Could you check a few things on this model? Use its own coordinates, in mm. A direction names the side the tool comes from. Round coordinates to 2 decimals unless told otherwise and drop trailing zeros. Loops run counter-clockwise (first coordinate to the right, second up) from the corner with the lowest first, then second, coordinate; pieces in that order, holes last. Notation, with made-up numbers: M 64.25,-14 L 112.25,-14 A18 ccw 112.25,-3 Z; hole C 24,-6 d8. An arc over 180 degrees is marked long. Return JSON: item names as keys, results as strings. Group by question number.
```python
from build123d import *

# Parameters (mm, degrees)
F0_R      = 3
F1_DEPTH  = 5
F2_DEPTH  = 10
F0_R_2    = 2
F3_DEPTH  = 8
F4_DEPTH  = 4
F6_DEPTH  = 4
F0_R_3    = 1
F7_DEPTH  = 6
F9_DEPTH  = 5
F10_DEPTH = 3
F12_DEPTH = 3


with BuildPart() as f1:
    # F0 (on Front) → F1 (new body)
    with BuildSketch(Plane.XZ):
        with BuildLine():
            Line((0, -35.3999999996), (2.6533119314, -35.3999999996))
            ThreePointArc((2.6533119314, -35.3999999996), (4.384153616, -33.1616546164), (5, -30.3999999996))
            ThreePointArc((5, -30.3999999996), (3.5355339059, -26.8644660937), (0, -25.3999999997))
            ThreePointArc((0, -25.3999999997), (-4.9999999999, -30.3999999996), (0, -35.3999999996))
        make_face()
        with Locations((0, -30.3999999996)):
            Circle(F0_R, mode=Mode.SUBTRACT)
    extrude(amount=F1_DEPTH)

    # F0 (on Front) → F2 (join)
    with BuildSketch(Plane.XZ):
        with BuildLine():
            Line((2.6533119314, -35.3999999996), (12.8845462929, -35.3999999996))
            Line((12.8845462929, -35.3999999996), (32.6248164724, -18.8359465726))
            Line((32.6248164724, -18.8359465726), (37.09957244, 6.5416555939))
            Line((37.09957244, 6.5416555939), (24.2150261472, 28.8583444057))
            Line((24.2150261472, 28.8583444057), (0, 37.6718931452))
            Line((0, 37.6718931452), (0, 25.3999999997))
            ThreePointArc((0, 25.3999999997), (5.2987193342, 24.841166909), (10.3642812115, 23.1892577491))
            Line((10.3642812115, 23.1892577491), (10.3642812115, 25.3641809438))
            ThreePointArc((10.3642812115, 25.3641809438), (6.2595477971, 26.6754205469), (2, 27.326909814))
            Line((2, 27.326909814), (2, 34.8155971317))
            Line((2, 34.8155971317), (22.8469455738, 27.2279294674))
            Line((22.8469455738, 27.2279294674), (35.0035513982, 6.1720705321))
            Line((35.0035513982, 6.1720705321), (30.7816065022, -17.7717688002))
            Line((30.7816065022, -17.7717688002), (12.1566058243, -33.3999999997))
            Line((12.1566058243, -33.3999999997), (6.3245553202, -33.3999999997))
            ThreePointArc((6.3245553202, -33.3999999997), (6.9899965839, -30.0259040815), (5.9682330797, -26.7421052628))
            Line((5.9682330797, -26.7421052628), (5.9682330797, -24.6888678131))
            ThreePointArc((5.9682330797, -24.6888678131), (3.0052252445, -25.2215903784), (0, -25.3999999997))
            ThreePointArc((0, -25.3999999997), (3.5355339059, -26.8644660937), (5, -30.3999999996))
            ThreePointArc((5, -30.3999999996), (4.384153616, -33.1616546164), (2.6533119314, -35.3999999996))
        make_face()
    extrude(amount=F2_DEPTH)

    # F0 (on Front) → F3 (join)
    with BuildSketch(Plane.XZ):
        with BuildLine():
            ThreePointArc((10.3642812115, 25.3641809438), (27.3030038884, -2.3034710008), (5.9682330797, -26.7421052628))
            ThreePointArc((5.9682330797, -26.7421052628), (6.9899965839, -30.0259040815), (6.3245553202, -33.3999999997))
            Line((6.3245553202, -33.3999999997), (12.1566058243, -33.3999999997))
            Line((12.1566058243, -33.3999999997), (30.7816065022, -17.7717688002))
            Line((30.7816065022, -17.7717688002), (35.0035513982, 6.1720705321))
            Line((35.0035513982, 6.1720705321), (22.8469455738, 27.2279294674))
            Line((22.8469455738, 27.2279294674), (2, 34.8155971317))
            Line((2, 34.8155971317), (2, 27.326909814))
            ThreePointArc((2, 27.326909814), (6.2595477971, 26.6754205469), (10.3642812115, 25.3641809438))
        make_face()
        with Locations((10.7639788756, -29.5737889045)):
            Circle(F0_R_2, mode=Mode.SUBTRACT)
        with Locations((27.2553512828, -15.7358844)):
            Circle(F0_R_2, mode=Mode.SUBTRACT)
        with Locations((30.9936419152, 5.4650153001)):
            Circle(F0_R_2, mode=Mode.SUBTRACT)
        with Locations((20.2296630396, 24.1087736043)):
            Circle(F0_R_2, mode=Mode.SUBTRACT)
        with Locations((30.9936419152, 5.4650153001)):
            Circle(F0_R_2)
        with Locations((27.2553512828, -15.7358844)):
            Circle(F0_R_2)
    extrude(amount=F3_DEPTH)

    # F0 (on Front) → F4 (join)
    with BuildSketch(Plane.XZ):
        with BuildLine():
            ThreePointArc((10.3642812115, 23.1892577491), (25.2936055675, -2.3223947512), (5.9682330797, -24.6888678131))
            Line((5.9682330797, -24.6888678131), (5.9682330797, -26.7421052628))
            ThreePointArc((5.9682330797, -26.7421052628), (27.3030038884, -2.3034710008), (10.3642812115, 25.3641809438))
            Line((10.3642812115, 25.3641809438), (10.3642812115, 23.1892577491))
        make_face()
    extrude(amount=F4_DEPTH)

    # F5 (on face) → F6 (join)
    with BuildSketch(Plane.XZ.offset(10)):
        with BuildLine():
            ThreePointArc((10.3642812115, 23.1892577491), (25.2936055675, -2.3223947512), (5.9682330797, -24.6888678131))
            Line((5.9682330797, -24.6888678131), (5.9682330797, -26.7421052628))
            ThreePointArc((5.9682330797, -26.7421052628), (27.3030038884, -2.3034710008), (10.3642812115, 25.3641809438))
            Line((10.3642812115, 25.3641809438), (10.3642812115, 23.1892577491))
        make_face()
    extrude(amount=-F6_DEPTH)

    # F0 (on Front) → F7 (join)
    with BuildSketch(Plane.XZ):
        with Locations((20.2296630396, 24.1087736043)):
            Circle(F0_R_2)
        with Locations((20.2296630396, 24.1087736043)):
            Circle(F0_R_3, mode=Mode.SUBTRACT)
        with Locations((10.7639788756, -29.5737889045)):
            Circle(F0_R_2)
        with Locations((10.7639788756, -29.5737889045)):
            Circle(F0_R_3, mode=Mode.SUBTRACT)
    extrude(amount=F7_DEPTH)

    # F8 (on face) → F9 (cut)
    with BuildSketch(Plane.XZ.offset(10)):
        with BuildLine():
            Line((2.6535725711, -35.3997834846), (4.1954981558, -35.3999999996))
            Line((4.1954981558, -35.3999999996), (4.5446208272, -33.4200269408))
            ThreePointArc((4.5446208272, -33.4200269408), (5.2048555211, -28.7618241261), (1.9956840643, -25.3214779407))
            ThreePointArc((1.9956840643, -25.3214779407), (0.9986141145, -25.3803618933), (0, -25.3999999997))
            ThreePointArc((0, -25.3999999997), (3.5355339059, -26.8644660937), (5, -30.3999999996))
            ThreePointArc((5, -30.3999999996), (4.9127701426, -31.4613100854), (4.6534218159, -32.4941346551))
            ThreePointArc((4.6534218159, -32.4941346551), (3.854365705, -34.0852093419), (2.6535725711, -35.3997834846))
        make_face()
        with BuildLine():
            Line((2.6533119314, -35.3999999996), (4.1954981558, -35.3999999996))
            Line((4.1954981558, -35.3999999996), (2.6535725711, -35.3997834846))
            ThreePointArc((2.6535725711, -35.3997834846), (2.6534422527, -35.3998917438), (2.6533119314, -35.3999999996))
        make_face()
        with BuildLine():
            Line((0.0760534773, -35.399421553), (2.6535725711, -35.3997834846))
            ThreePointArc((2.6535725711, -35.3997834846), (3.854365705, -34.0852093419), (4.6534218159, -32.4941346551))
            ThreePointArc((4.6534218159, -32.4941346551), (4.9127701426, -31.4613100854), (5, -30.3999999996))
            ThreePointArc((5, -30.3999999996), (3.5623213911, -33.9085419057), (0.0760534773, -35.399421553))
        make_face()
        with BuildLine():
            ThreePointArc((0, -25.3999999997), (0.9986141145, -25.3803618933), (1.9956840643, -25.3214779407))
            ThreePointArc((1.9956840643, -25.3214779407), (1.0155877723, -25.0387760102), (0, -24.943431372))
            Line((0, -24.943431372), (0, -25.3999999997))
        make_face()
    extrude(amount=-F9_DEPTH, mode=Mode.SUBTRACT)

    # F0 (on Front) → F10 (cut)
    with BuildSketch(Plane.XZ):
        with Locations((20.2296630396, 24.1087736043)):
            Circle(F0_R_2)
        with Locations((20.2296630396, 24.1087736043)):
            Circle(F0_R_3, mode=Mode.SUBTRACT)
        with Locations((10.7639788756, -29.5737889045)):
            Circle(F0_R_2)
        with Locations((10.7639788756, -29.5737889045)):
            Circle(F0_R_3, mode=Mode.SUBTRACT)
    extrude(amount=F10_DEPTH, mode=Mode.SUBTRACT)

    # F11 (on face) → F12 (cut)
    with BuildSketch(Plane.XZ):
        with BuildLine():
            Line((8.3644706756, 32.4991192489), (2, 34.8155971317))
            Line((2, 34.8155971317), (2, 27.326909814))
            ThreePointArc((2, 27.326909814), (5.2188864899, 26.8983870108), (8.3644706756, 26.0920606756))
            Line((8.3644706756, 26.0920606756), (8.3644706756, 32.4991192489))
        make_face()
    extrude(amount=F12_DEPTH, mode=Mode.SUBTRACT)


solid = f1.part
```
1. On a 3-axis mill with a long thin cutter (end or side, diameter ignored), from which of +Z, -Z, +X, -X, +Y, -Y can I reach the whole of each face in a straight line? I mean faces 5 (the face through (18.643, -1.479, 22.892)), 6 (the face through (27.34, -4.99, -1.82)), 7 (the face through (19, -6, 24)). Say none if no direction works.
2. We'd pull the mould along X, two halves only. Please class faces 1 (the face through (5.23, -1.48, 33.64)), 2 (the face through (8, -5, -35.4)), 3 (the face through (5.225, -7.535, -28.827)), 4 (the face through (8.364, -1, 29)): +X half, -X half, draft (parallel to the pull), parting line (faces both ways), or undercut.
3. If we section it at B-B, the plane x = 26.5: Please give me the cut outline in (y, z).
4. If we section it at D-D, the plane z = 7.5: Please give me the cut outline in (x, y).
5. If we section it at A-A, the plane y = -7: Please give me the cut outline in (x, z).
6. If we section it at C-C, the plane y = -1.75: Please give me the cut outline in (x, z).
7. I need wall thicknesses on probe 1 along Y at (x, z) = (25.5, -7); probe 2 along Z at (x, y) = (12.5, -7); probe 3 along Y at (x, z) = (4, -31). Which ranges of each line are inside material? Lowest first, please.
8. I'm going to push flat-ended pins straight in: pin 1 Ø4.5 at (x, z) = (20.23, 24.11) entering from +Y; pin 2 Ø4 at (y, z) = (-7, 1) entering from +X; pin 3 Ø3 at (x, z) = (0.5, -32) entering from -Y; pin 4 Ø3 at (x, z) = (20.23, 24.11) entering from -Y. Where does each tip first touch, or does it pass through?
Geometry results:
{
 "1": {"face 5": "+Y", "face 6": "none", "face 7": "-Y"},
 "2": {"face 1": "undercut", "face 2": "draft", "face 3": "-X half", "face 4": "undercut"},
 "3": {"outline": "M -10,-23.98 L 0,-23.98 L 0,24.9 L -10,24.9 L -10,20.9 L -8,20.9 L -8,6.96 L -10,6.96 L -10,-6.96 L -8,-6.96 L -8,-21.36 L -10,-21.36 Z; hole M -6,-6.96 L -4,-6.96 L -4,6.96 L -6,6.96 Z"},
 "4": {"outline": "M 24.27,-10 L 26.35,-10 L 26.35,-8 L 34.24,-8 L 34.24,-10 L 36.55,-10 L 36.55,0 L 24.27,0 L 24.27,-4 L 26.35,-4 L 26.35,-6 L 24.27,-6 Z"},
 "5": {"outline": "M 0,25.4 A25.4 cw 2,-25.32 A5.46 cw 4.54,-33.42 L 4.2,-35.4 L 12.88,-35.4 L 32.62,-18.84 L 37.1,6.54 L 24.22,28.86 L 0,37.67 Z; hole C 10.76,-29.57 d4; hole C 20.23,24.11 d4"},
 "6": {"outline": "M 0,-35.4 L 12.88,-35.4 L 32.62,-18.84 L 37.1,6.54 L 24.22,28.86 L 0,37.67 L 0,25.4 A25.4 cw 0,-25.4 A5 ccw Z; hole C 0,-30.4 d6; hole M 2,27.33 A27.4 cw 8.36,26.09 L 8.36,32.5 L 2,34.82 Z; hole C 10.76,-29.57 d4; hole C 20.23,24.11 d4"},
 "7": {"probe 1": "-10 to -6, -4 to 0", "probe 2": "-35.4 to -30.57, -28.58 to -22.11, 22.11 to 33.12", "probe 3": "-5 to 0"},
 "8": {"pin 1": "y = 0", "pin 2": "x = 36.48", "pin 3": "y = -5", "pin 4": "y = -6"}
}
